Read the model definition and answer for the solid it produces. Units are mm, in the model's axes. A direction names the side the tool comes from. Give positions to 0.01 mm unless a question says otherwise; leave off trailing zeros. Write each loop counter-clockwise with the first axis right and the second up, starting at its lowest first coordinate (ties: lowest second). Pieces come first, ordered by that corner, then holes. Notation, with made-up numbers: (26, 45.25) - (78, 45.25) arc R24 cw to (78, 68.25) - close; hole circle Ø1 at (67, 79). An arc over 180 degrees is marked (long way). Answer as a JSON object with one key per item and string values. Group by question number.
```python
from build123d import *

# Parameters (mm, degrees)
BOSS_EXTRUDE1_DEPTH = 8
BOSS_EXTRUDE2_DEPTH = 8


with BuildPart() as part:
    # Sketch2 → Boss-Extrude1 (new body)
    with BuildSketch(Plane(origin=(0, 0, 0), x_dir=(0, 0, -1), z_dir=(1, 0, 0))):
        Polygon((-10.928495294, -9.782945939), (25.071504706, -9.782945939), (25.071504706, -3.782945939), (-10.928495294, 9.319982495), align=None)
    extrude(amount=-BOSS_EXTRUDE1_DEPTH)

    # Cut-Sweep3: sweep along a path in Sketch5
    with BuildLine(Plane.ZY.offset(8)) as cut_sweep3_path:
        Line((-25.071504706, -6.975479256), (8.757429642, 5.337245904))
    # Sketch3 → Cut-Sweep3 (sweep, cut)
    with BuildSketch(Plane(origin=(0, 0, -25.071504706), x_dir=(-1, 0, 0), z_dir=(0, 0, -1))):
        Polygon((2.875, -3.782945939), (2.875, -4.782945939), (1, -4.782945939), (1, -6.782945939), (7, -6.782945939), (7, -4.782945939), (5.125, -4.782945939), (5.125, -3.782945939), align=None)
    sweep(path=cut_sweep3_path.line, mode=Mode.SUBTRACT)

    # Sketch6 → Boss-Extrude2 (add)
    with BuildSketch(Plane.ZY.offset(8)):
        Polygon((4.906861068, 3.935753558), (8.195785241, 5.132824059), (5.117603951, 13.590057646), (1.828679778, 12.392987145), align=None)
    extrude(amount=-BOSS_EXTRUDE2_DEPTH)


solid = part.part
```
1) Find the intervals of material crossed by line 1 (Z direction, x = -5, y = 5.75); line 2 (X direction, y = 2.5, z = -2.5); line 3 (Y direction, x = -6.25, z = -2.5), in increasing order. Write a range as [from, to].
2) Find section A-A, the plane x = -1.75. Write down the section's boundary in (y, z), and give its area (3 significant figures).
3) Find section B-B, the plane x = -4.5. Write down the section's boundary in (y, z), and give its area (3 significant figures).
4) Flat-ended cylindrical pins translate along their axes: pin 1 Ø6 at (y, z) = (3.5, -17) entering from +X; pin 2 Ø1 at (x, y) = (-1.5, 10.5) entering from -Z; pin 3 Ø1.5 at (x, y) = (-3.5, 7.5) entering from -Z. Find the tip coordinate at first contact, or state that the pin passes through.
5) For a pull along X with two mould halves and no side action, classify faces 1 (the flat face through (0, -3, -3)), 2 (the flat face through (-4.1, 13, 3.5)), 3 (the flat face through (-1, 6.4, 8.3)) as released by +X, released by -X, zero draft, split by the parting line, or undercut.
6) Which of the six approach directions +Z, -Z, +X, -X, +Y, -Y give full straight-line access (tool end or side, diameter ignored) to faces 4 (the flat face through (-5.125, 8, 8)), 5 (the flat face through (-4, -7, -25.072)), 6 (the flat face through (-1, 0, -10))?
7) Find section D-D, the plane y = -5.75. Write down the section's boundary in (x, z).
8) Find section C-C, the plane z = -22.5. Write down the section's boundary in (x, y) (3 decimals).
Values follow:
{
 "1": {"line 1": "z = [4.25, 7.97], [8.76, 10.93]", "line 2": "x = [-8, -7], [-1, 0]", "line 3": "y = [-9.78, 1.43], [3.43, 4.43]"},
 "2": {"outline": "(-9.78, -25.07) - (-6.78, -25.07) - (4.11, 4.84) - (5.87, 4.2) - (-4.78, -25.07) - (-3.78, -25.07) - (6.75, 3.88) - (12.39, 1.83) - (13.59, 5.12) - (7.95, 7.17) - (9.32, 10.93) - (-9.78, 10.93) - close; hole (5.3, 8.13) - (7.07, 7.49) - (7.53, 8.76) - (5.53, 8.76) - close", "area": "412 mm2"},
 "3": {"outline": "(-9.78, -25.07) - (-6.78, -25.07) - (4.11, 4.84) - (12.39, 1.83) - (13.59, 5.12) - (5.3, 8.13) - (5.53, 8.76) - (8.53, 8.76) - (9.32, 10.93) - (-9.78, 10.93) - close", "area": "381 mm2"},
 "4": {"pin 1": "passes through", "pin 2": "stops at z = 2.34", "pin 3": "stops at z = 3.34"},
 "5": {"face 1": "released by +X", "face 2": "zero draft", "face 3": "undercut"},
 "6": {"face 4": "+Y", "face 5": "-Z, +X, -X, +Y, -Y", "face 6": "none"},
 "7": {"outline": "(-8, -25.07) - (-7, -25.07) - (-7, -22.23) - (-1, -22.23) - (-1, -25.07) - (0, -25.07) - (0, 10.93) - (-8, 10.93) - close"},
 "8": {"outline": "(-8, -9.783) - (0, -9.783) - (0, -2.847) - (-2.875, -2.847) - (-2.875, -3.847) - (-1, -3.847) - (-1, -5.847) - (-7, -5.847) - (-7, -3.847) - (-5.125, -3.847) - (-5.125, -2.847) - (-8, -2.847) - close"}
}
